CAD build for the part. Positions are in the model's coordinates, mm. A direction names the side the tool comes from. Give positions to 0.01 mm unless a question says otherwise; leave off trailing zeros. Order: outer loops, then holes, each group sorted by start corner. A loop starts at its lowest first (then second) coordinate and runs counter-clockwise, first axis right, second up.
from build123d import *

# Parameters (mm, degrees)
BOSS_EXTRU_1_DEPTH      = 5
ESQUISSE3_R             = 3
ESQUISSE3_W             = 5
ESQUISSE3_H             = 48.75
ESQUISSE3_H_2           = 3.25
ESQUISSE3_H_3           = 10
ESQUISSE3_W_2           = 9
ESQUISSE3_H_4           = 5
ENL_V_MAT_EXTRU_1_DEPTH = 5
ESQUISSE4_W             = 10
ESQUISSE4_H             = 5
ESQUISSE4_W_2           = 15
ESQUISSE4_W_3           = 5
BOSS_EXTRU_2_DEPTH      = 5
ESQUISSE5_R             = 1.5
ENL_V_MAT_EXTRU_2_DEPTH = 5


with BuildPart() as part:
    # Esquisse1 → Boss.-Extru.1 (new body)
    with BuildSketch(Plane.XY):
        with BuildLine():
            Line((0, 0), (29, 0))
            Line((29, 0), (30.512421766, 31.797613203))
            ThreePointArc((30.512421766, 31.797613203), (41.5, 42.275), (52.487578234, 31.797613203))
            Line((52.487578234, 31.797613203), (54, 0))
            Line((54, 0), (83, 0))
            Line((83, 0), (83, 73))
            Line((83, 73), (0, 73))
            Line((0, 73), (0, 0))
        make_face()
    extrude(amount=BOSS_EXTRU_1_DEPTH)

    # Esquisse3 → Enlèv. mat.-Extru.1 (cut)
    with BuildSketch(Plane.XY.offset(5)):
        with Locations((41.5, 44.275)):
            Circle(ESQUISSE3_R)
        with Locations((54.5, 31.275)):
            Circle(ESQUISSE3_R)
        with Locations((28.5, 31.275)):
            Circle(ESQUISSE3_R)
        Polygon((15, 73), (0, 73), (0, 67), (5, 67), (5, 68), (15, 68), align=None)
        Polygon((78, 67), (83, 67), (83, 73), (68, 73), (68, 68), (78, 68), align=None)
        with Locations((2.5, 32.625)):
            Rectangle(ESQUISSE3_W, ESQUISSE3_H)
        with Locations((2.5, 1.625)):
            Rectangle(ESQUISSE3_W, ESQUISSE3_H_2)
        with Locations((80.5, 1.625)):
            Rectangle(ESQUISSE3_W, ESQUISSE3_H_2)
        with Locations((80.5, 32.625)):
            Rectangle(ESQUISSE3_W, ESQUISSE3_H)
        with Locations((62, 15)):
            Rectangle(ESQUISSE3_W, ESQUISSE3_H_3)
        with Locations((21, 53)):
            Rectangle(ESQUISSE3_W, ESQUISSE3_H_3)
        with Locations((21, 15)):
            Rectangle(ESQUISSE3_W, ESQUISSE3_H_3)
        with Locations((62, 53)):
            Rectangle(ESQUISSE3_W, ESQUISSE3_H_3)
        with Locations((53.5, 70.5)):
            Rectangle(ESQUISSE3_W_2, ESQUISSE3_H_4)
        with Locations((29.5, 70.5)):
            Rectangle(ESQUISSE3_W_2, ESQUISSE3_H_4)
    extrude(amount=-ENL_V_MAT_EXTRU_1_DEPTH, mode=Mode.SUBTRACT)

    # Esquisse4 → Boss.-Extru.2 (add)
    with BuildSketch(Plane(origin=(0, 0, 0), x_dir=(-1, 0, 0), z_dir=(0, 0, -1))):
        with Locations((-63, 75.5)):
            Rectangle(ESQUISSE4_W, ESQUISSE4_H)
        with Locations((-41.5, 75.5)):
            Rectangle(ESQUISSE4_W_2, ESQUISSE4_H)
        with Locations((-20, 75.5)):
            Rectangle(ESQUISSE4_W, ESQUISSE4_H)
        with Locations((-75.5, -2.5)):
            Rectangle(ESQUISSE4_W_3, ESQUISSE4_H)
        with Locations((-7.5, -2.5)):
            Rectangle(ESQUISSE4_W_3, ESQUISSE4_H)
    extrude(amount=-BOSS_EXTRU_2_DEPTH)

    # Esquisse5 → Enlèv. mat.-Extru.2 (cut)
    with BuildSketch(Plane.XY.offset(5)):
        with Locations((52.5, 46.275)):
            Circle(ESQUISSE5_R)
        with Locations((30.5, 46.275)):
            Circle(ESQUISSE5_R)
    extrude(amount=-ENL_V_MAT_EXTRU_2_DEPTH, mode=Mode.SUBTRACT)


solid = part.part
1. Saw through at C-C on x = 75. Give the cut face in (y, z), plus the area to 3 significant figures.
2. Saw through at D-D on z = 2.85. State how many separate pieces and enclosed holes the cut face has, plus the area to 3 significant figures.
3. 3-axis set-ups, long thin cutter, end or side, ignore diameter. For faces 5 (the cylindrical face through (49.21, 39.12, 2.46)), 6 (the flat face through (78, 32, 3)), 7 (the flat face through (23.5, 53, 3)), 8 (the flat face through (2, 8.25, 3)): which of +Z, -Z, +X, -X, +Y, -Y reach the whole face in a straight line?
4. Pin check, flat tips, straight feed: P1, Ø2.5, axis at x = 3, z = 1.5, coming from the +Y side; P2, Ø0.8, axis at y = 67.5, z = 1.5, coming from the -X side; P3, Ø1.5, axis at x = 21.5, z = 2, coming from the -Y side. Stop position of each tip, or through.
5. Mould opens along X. For faces 1 (the flat face through (2, 67, 3)), 2 (the cylindrical face through (57.498, 31.393, 2.535)), 3 (the flat face through (68, 73, 2)), 4 (the flat face through (21, 10, 3)) say: released by +X, released by -X, zero draft, split by the parting line, or undercut.
6. Wall check: line 1 (Y direction, x = 61, z = 4.35); line 2 (X direction, y = 50, z = 4.05); line 3 (Y direction, x = 54.5, z = 2.35) (3 decimals). Give the ranges that are in metal, low to high.
7. Saw through at B-B on y = 37.5. Give the cut face in (x, z), plus the area to 3 significant figures.
8. Saw through at A-A on y = 18.5. Give the cut face in (x, z), plus the area to 3 significant figures.
Reported:
1. outline: (-5, 0) - (68, 0) - (68, 5) - (-5, 5) - close
1. area: 365 mm2
2. separate pieces: 1
2. enclosed holes: 6
2. area: 4,300 mm2
3. face 5: +Z, -Z, -Y
3. face 6: +Z, -Z, +X
3. face 7: +Z, -Z
3. face 8: +Z, -Z, -X
4. P1: stops at y = 67
4. P2: stops at x = 5
4. P3: stops at y = 0
5. face 1: zero draft
5. face 2: undercut
5. face 3: released by +X
5. face 4: undercut
6. line 1: y = 0 to 10, 20 to 48, 58 to 78
6. line 2: x = 5 to 18.5, 23.5 to 59.5, 64.5 to 78
6. line 3: y = 0 to 28.275, 34.275 to 68
7. outline: (5, 0) - (32.43, 0) - (32.43, 5) - (5, 5) - close; (50.57, 0) - (78, 0) - (78, 5) - (50.57, 5) - close
7. area: 274 mm2
8. outline: (5, 0) - (18.5, 0) - (18.5, 5) - (5, 5) - close; (23.5, 0) - (29.88, 0) - (29.88, 5) - (23.5, 5) - close; (53.12, 0) - (59.5, 0) - (59.5, 5) - (53.12, 5) - close; (64.5, 0) - (78, 0) - (78, 5) - (64.5, 5) - close
8. area: 199 mm2
